Read the model definition and answer for the solid it produces. Units are mm, in the model's axes. Face numbers are marked on the shaded views. A direction names the side the tool comes from. Round coordinates to 2 decimals unless told otherwise and drop trailing zeros. Loops run counter-clockwise (first coordinate to the right, second up) from the corner with the lowest first, then second, coordinate; pieces in that order, holes last. Notation, with made-up numbers: M -34.5,59.25 L 15.5,59.25 A11 cw 15.5,68.25 Z; hole C 4.25,84 d1. An arc over 180 degrees is marked long. Write each question's results on one line, items separated by ' | '.
```python
from build123d import *

# Parameters (mm, degrees)
F0_W     = 10
F0_H     = 50
F1_DEPTH = 10
F2_R     = 2.5
F3_DEPTH = 10


with BuildPart() as f1:
    # F0 (on Front) → F1 (new body)
    with BuildSketch(Plane.XZ):
        Rectangle(F0_W, F0_H)
        Polygon((5, -35), (5, -25), (-5, -25), (-25, -25), (-25, -35), align=None)
    extrude(amount=F1_DEPTH)

    # F2 (on face) → F3 (cut, through all)
    with BuildSketch(Plane.XZ.offset(10)):
        with Locations((0, 20)):
            Circle(F2_R)
    extrude(amount=-F3_DEPTH, mode=Mode.SUBTRACT)


solid = f1.part
```
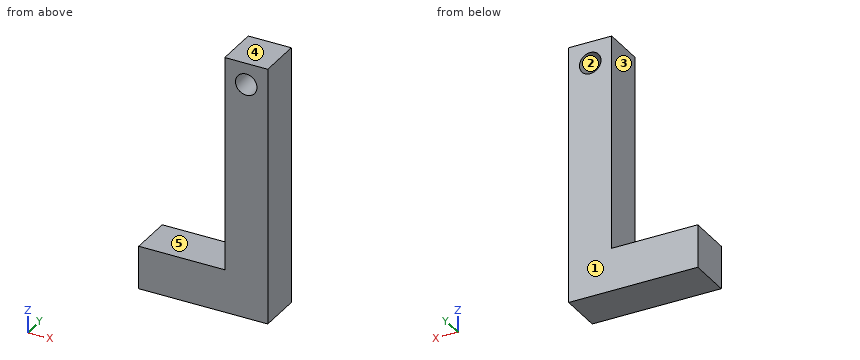
1. Which of the six approach directions +Z, -Z, +X, -X, +Y, -Y give full straight-line access (tool end or side, diameter ignored) to the marked faces 4 and 5?
Completed:
face 4: +Z, +X, -X, +Y, -Y | face 5: +Z, -X, +Y, -Y
2. Find section B-B, the plane x = 0. Give the vertices of the cut face in (y, z).
Completed:
outline: M -10,-35 L 0,-35 L 0,17.5 L -10,17.5 Z; M -10,22.5 L 0,22.5 L 0,25 L -10,25 Z
3. Determine the mould class of the marked faces 1, 2 and 3 for opening direction X: released by +X, released by -X, zero draft, split by the parting line, or undercut.
Completed:
face 1: zero draft | face 2: undercut | face 3: released by -X
4. Find section C-C, the plane y = -1.25. Give the vertices of the cut face in (x, z).
Completed:
outline: M -25,-35 L 5,-35 L 5,25 L -5,25 L -5,-25 L -25,-25 Z; hole C 0,20 d5
5. Find the intervals of material crossed by L1, parallel to Z at x = 0, y = -6; L2, parallel to X at y = -2, z = 6; L3, parallel to Z at x = -17.75, y = -7, in increasing order.
Completed:
L1: z = -35 to 17.5, 22.5 to 25 | L2: x = -5 to 5 | L3: z = -35 to -25
6. Given P1, Ø3, axis at x = -17, y = -3, coming from the +Z side; P2, Ø1, axis at y = -8, z = 12, coming from the -X side, each flat-ended and moving along its own axis, determine where each tip first touches the part or whether it passes through.
Completed:
P1: stops at z = -25 | P2: stops at x = -5
7. Find section A-A, the plane z = 20. Give the vertices of the cut face in (x, y), then the cut area to 3 significant figures.
Completed:
outline: M -5,-10 L -2.5,-10 L -2.5,0 L -5,0 Z; M 2.5,-10 L 5,-10 L 5,0 L 2.5,0 Z | area: 50.0 mm2
8. Find section D-D, the plane z = -11.5. Give the vertices of the cut face in (x, y), then the cut area to 3 significant figures.
Completed:
outline: M -5,-10 L 5,-10 L 5,0 L -5,0 Z | area: 100 mm2
